The model under review builds one solid part; all positions refer to its coordinate system, in mm. A direction names the side the tool comes from. Coordinates: 2 decimals unless noted, no trailing zeros. Write each loop counter-clockwise with the first axis right and the second up, starting at its lowest first coordinate (ties: lowest second). Pieces come first, ordered by that corner, then holes.
```python
from build123d import *

# Parameters (mm, degrees)
F0_W     = 200
F0_H     = 200
F1_DEPTH = 70
F2_T     = -2
F3_W     = 2
F3_H     = 196
F4_DEPTH = 68


with BuildPart() as f1:
    # F0 (on Top) → F1 (new body)
    with BuildSketch(Plane.XY):
        with Locations((-7.9974851012, -33.8844692809)):
            Rectangle(F0_W, F0_H)
    extrude(amount=F1_DEPTH)

    # F2
    f2_openings = [f1.faces().sort_by_distance(p)[0] for p in [
        (-7.997485, -33.884469, 70),
    ]]
    offset(amount=F2_T, openings=f2_openings)

    # F3 (on face) → F4 (join)
    with BuildSketch(Plane.XY.offset(2)):
        with Locations((-54.9974851012, -33.8844692809)):
            Rectangle(F3_W, F3_H)
        with Locations((-2.9974851012, -33.8844692809)):
            Rectangle(F3_W, F3_H)
        with Locations((44.0025148988, -33.8844692809)):
            Rectangle(F3_W, F3_H)
    extrude(amount=F4_DEPTH)


solid = f1.part
```
Item 1: Take a section at B-B, the plane z = 24.5. Write out the cut boundary in (x, y), plus the area to 3 significant figures.
Solved:
outline: (-108, -133.88) - (92, -133.88) - (92, 66.12) - (-108, 66.12) - close; hole (-106, -131.88) - (-56, -131.88) - (-56, 64.12) - (-106, 64.12) - close; hole (-54, -131.88) - (-4, -131.88) - (-4, 64.12) - (-54, 64.12) - close; hole (-2, -131.88) - (43, -131.88) - (43, 64.12) - (-2, 64.12) - close; hole (45, -131.88) - (90, -131.88) - (90, 64.12) - (45, 64.12) - close
area: 2,760 mm2
Item 2: To check wall thickness, follow line 1 along X through (y, z) = (-55.5, 41); line 2 along Y through (x, z) = (5, 56); line 3 along Z through (x, y) = (-92.5, -34.5). State the ranges of each line that lie inside material, in increasing order.
Solved:
line 1: x = -108 to -106, -56 to -54, -4 to -2, 43 to 45, 90 to 92
line 2: y = -133.88 to -131.88, 64.12 to 66.12
line 3: z = 0 to 2
Item 3: For pin 1 (13.5 mm diameter, centred on x = 57.5, y = -36.5, fed in from +Z), flat-tipped, find the tip position at first contact; note if it passes through.
Solved:
pin 1: stops at z = 2
Item 4: Take a section at C-C, the plane x = -80.5. Write out the cut boundary in (y, z), plus the area to 3 significant figures.
Solved:
outline: (-133.88, 0) - (66.12, 0) - (66.12, 70) - (64.12, 70) - (64.12, 2) - (-131.88, 2) - (-131.88, 70) - (-133.88, 70) - close
area: 672 mm2
Item 5: Machinability: for faces 1 (the face through (92.003, -35, 35)), 2 (the face through (67, -33, 2)), which of the approach directions +Z, -Z, +X, -X, +Y, -Y give a long, thin tool a straight path to every point of the face, cutting with its end or side? Answer none if there is none.
Solved:
face 1: +Z, -Z, +X, +Y, -Y
face 2: +Z
Item 6: Take a section at A-A, the plane y = -69. Write out the cut boundary in (x, z), plus the area to 3 significant figures.
Solved:
outline: (-108, 0) - (92, 0) - (92, 70) - (90, 70) - (90, 2) - (45, 2) - (45, 70) - (43, 70) - (43, 2) - (-2, 2) - (-2, 70) - (-4, 70) - (-4, 2) - (-54, 2) - (-54, 70) - (-56, 70) - (-56, 2) - (-106, 2) - (-106, 70) - (-108, 70) - close
area: 1,080 mm2
Item 7: Mouldability with a two-part tool opening along Y and no side actions: class faces 3 (the face through (-29, -33, 2)), 4 (the face through (-81, 64.116, 36)), 5 (the face through (-9, 66.116, 35)), 6 (the face through (-107.997, -35, 35)) as pulls with the +Y half, pulls with the -Y half, needs draft (parallel to the pull), parting line crosses it, or undercut.
Solved:
face 3: undercut
face 4: undercut
face 5: pulls with the +Y half
face 6: needs draft
